from build123d import *

# Parameters (mm, degrees)
BOSS_EXTRUDE1_DEPTH = 3.175
CUT_EXTRUDE1_REACH  = 5.175
SKETCH2_R           = 1.4
SKETCH2_R_2         = 2
SKETCH2_R_3         = 2.876999961
CUT_EXTRUDE2_DEPTH  = 4.175


with BuildPart() as part:
    # Sketch1 → Boss-Extrude1 (new body)
    with BuildSketch(Plane(origin=(0, 0, 0), x_dir=(0, 0, -1), z_dir=(1, 0, 0))):
        Polygon((0, 0), (0, 59.6392), (12.7, 59.6392), (12.7, 57.15), (25.4, 57.15), (25.4, 59.6392), (38.1, 59.6392), (38.1, 57.15), (50.8, 57.15), (50.8, 59.6392), (63.5, 59.6392), (63.5, 57.15), (76.2, 57.15), (76.2, 59.6392), (88.9, 59.6392), (88.9, 57.15), (101.6, 57.15), (101.6, 0), align=None)
    extrude(amount=BOSS_EXTRUDE1_DEPTH)

    # Sketch2 → Cut-Extrude1 (cut, up to next)
    with BuildSketch(Plane(origin=(3.175, 0, 0), x_dir=(0, 0, -1), z_dir=(1, 0, 0)), mode=Mode.PRIVATE) as cut_extrude1_sk1:
        with Locations((30.59102, 10.3)):
            Circle(SKETCH2_R)
    cut_extrude1_tool1 = extrude(cut_extrude1_sk1.sketch, amount=-CUT_EXTRUDE1_REACH, mode=Mode.PRIVATE) & part.part
    add(cut_extrude1_tool1.solids().sort_by_distance((3.175, 10.3, -30.59102))[0], mode=Mode.SUBTRACT)
    # Sketch2 → Cut-Extrude1 (cut, up to next)
    with BuildSketch(Plane(origin=(3.175, 0, 0), x_dir=(0, 0, -1), z_dir=(1, 0, 0)), mode=Mode.PRIVATE) as cut_extrude1_sk2:
        with Locations((30.59102, 27.8)):
            Circle(SKETCH2_R)
    cut_extrude1_tool2 = extrude(cut_extrude1_sk2.sketch, amount=-CUT_EXTRUDE1_REACH, mode=Mode.PRIVATE) & part.part
    add(cut_extrude1_tool2.solids().sort_by_distance((3.175, 27.8, -30.59102))[0], mode=Mode.SUBTRACT)
    # Sketch2 → Cut-Extrude1 (cut, up to next)
    with BuildSketch(Plane(origin=(3.175, 0, 0), x_dir=(0, 0, -1), z_dir=(1, 0, 0)), mode=Mode.PRIVATE) as cut_extrude1_sk3:
        with Locations((22.0000034, 19.05)):
            Circle(SKETCH2_R_2)
    cut_extrude1_tool3 = extrude(cut_extrude1_sk3.sketch, amount=-CUT_EXTRUDE1_REACH, mode=Mode.PRIVATE) & part.part
    add(cut_extrude1_tool3.solids().sort_by_distance((3.175, 19.05, -22.000003))[0], mode=Mode.SUBTRACT)
    # Sketch2 → Cut-Extrude1 (cut, up to next)
    with BuildSketch(Plane(origin=(3.175, 0, 0), x_dir=(0, 0, -1), z_dir=(1, 0, 0)), mode=Mode.PRIVATE) as cut_extrude1_sk4:
        with Locations((11, 19.05)):
            Circle(SKETCH2_R_3)
    cut_extrude1_tool4 = extrude(cut_extrude1_sk4.sketch, amount=-CUT_EXTRUDE1_REACH, mode=Mode.PRIVATE) & part.part
    add(cut_extrude1_tool4.solids().sort_by_distance((3.175, 19.05, -11))[0], mode=Mode.SUBTRACT)

    # Sketch3 → Cut-Extrude2 (cut, through all)
    with BuildSketch(Plane(origin=(3.175, 0, 0), x_dir=(0, 0, -1), z_dir=(1, 0, 0))):
        Polygon((12.7, 57.15), (12.7, 59.6392), (12.573, 59.6392), (12.573, 57.023), (25.527, 57.023), (25.527, 59.6392), (25.4, 59.6392), (25.4, 57.15), align=None)
        Polygon((38.1, 59.6392), (37.973, 59.6392), (37.973, 57.023), (50.927, 57.023), (50.927, 59.6392), (50.8, 59.6392), (50.8, 57.15), (38.1, 57.15), align=None)
        Polygon((63.5, 59.6392), (63.373, 59.6392), (63.373, 57.023), (76.327, 57.023), (76.327, 59.6392), (76.2, 59.6392), (76.2, 57.15), (63.5, 57.15), align=None)
        Polygon((88.9, 59.6392), (88.773, 59.6392), (88.773, 57.023), (101.6, 57.023), (101.6, 57.15), (88.9, 57.15), align=None)
    extrude(amount=-CUT_EXTRUDE2_DEPTH, mode=Mode.SUBTRACT)


solid = part.part
CAD build for the part. Positions are in the model's coordinates, mm. A direction names the side the tool comes from. Give positions to 0.01 mm unless a question says otherwise; leave off trailing zeros. Loops run counter-clockwise (first coordinate to the right, second up) from the corner with the lowest first, then second, coordinate; pieces in that order, holes last. Notation, with made-up numbers: M -13,-12 L 41,-12 A22 ccw 41,4 Z; hole C -22,49.25 d11. An arc over 180 degrees is marked long. Answer in a Markdown table with one row per item. Add a question column.
Item 1: Band-saw the part on D-D on x = 1.05. Give the cut face in (y, z).
Item 2: Probe probe 1 along Y at (x, z) = (1.7, -11); probe 2 along Y at (x, z) = (3, -18); probe 3 along Y at (x, z) = (0.8, -21.5). List the from-to ranges inside material, lowest first.
Item 3: Band-saw the part on B-B on z = -11. Give the cut face in (x, y) (3 decimals).
Item 4: Tool access for faces 1 (the face through (2, 57.023, -95)), 2 (the face through (2, 57.023, -19)), 3 (the face through (1.6, 9.8, -31.9)): list every direction of +Z, -Z, +X, -X, +Y, -Y with a clear straight run to the whole face (end or side of a thin tool).
Item 5: Mould opens along Z. For faces 4 (the face through (2, 59.639, -6)), 5 (the face through (2, 57.023, -44)), 6 (the face through (2, 29, 0)) say: +Z half, -Z half, draft (parallel to the pull), parting line (faces both ways), or undercut.
Item 6: Band-saw the part on C-C on y = 10.3. Give the cut face in (x, z) (3 decimals).
Item 7: Drop flat-ended pins along their axis: P1, Ø1, axis at x = 2.5, z = -69, coming from the +Y side; P2, Ø0.8, axis at x = 1.5, y = 58, coming from the -Z side. Give the stop position or say it passes through.
Item 8: Band-saw the part on A-A on y = 19.05. Give the cut face in (x, z) (3 decimals).
Reply:
| question | item | result |
|---|---|---|
| 1 | outline | M 0,-101.6 L 57.02,-101.6 L 57.02,-88.77 L 59.64,-88.77 L 59.64,-76.33 L 57.02,-76.33 L 57.02,-63.37 L 59.64,-63.37 L 59.64,-50.93 L 57.02,-50.93 L 57.02,-37.97 L 59.64,-37.97 L 59.64,-25.53 L 57.02,-25.53 L 57.02,-12.57 L 59.64,-12.57 L 59.64,0 L 0,0 Z; hole C 10.3,-30.59 d2.8; hole C 19.05,-11 d5.75; hole C 19.05,-22 d4; hole C 27.8,-30.59 d2.8 |
| 2 | probe 1 | y = 0 to 16.17, 21.93 to 59.64 |
| 2 | probe 2 | y = 0 to 57.02 |
| 2 | probe 3 | y = 0 to 17.11, 20.99 to 57.02 |
| 3 | outline | M 0,0 L 3.175,0 L 3.175,16.173 L 0,16.173 Z; M 0,21.927 L 3.175,21.927 L 3.175,59.639 L 0,59.639 Z |
| 4 | face 1 | -Z, +X, -X, +Y |
| 4 | face 2 | +X, -X, +Y |
| 4 | face 3 | +X, -X |
| 5 | face 4 | draft |
| 5 | face 5 | undercut |
| 5 | face 6 | +Z half |
| 6 | outline | M 0,-101.6 L 3.175,-101.6 L 3.175,-31.991 L 0,-31.991 Z; M 0,-29.191 L 3.175,-29.191 L 3.175,0 L 0,0 Z |
| 7 | P1 | stops at y = 57.02 |
| 7 | P2 | stops at z = -88.77 |
| 8 | outline | M 0,-101.6 L 3.175,-101.6 L 3.175,-24 L 0,-24 Z; M 0,-20 L 3.175,-20 L 3.175,-13.877 L 0,-13.877 Z; M 0,-8.123 L 3.175,-8.123 L 3.175,0 L 0,0 Z |
